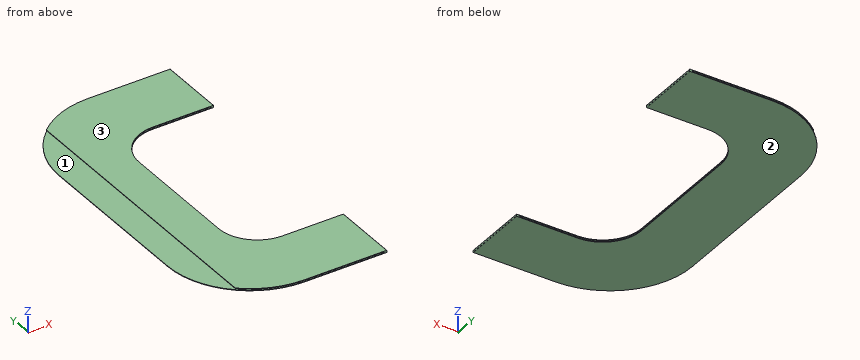
```python
from build123d import *

# Parameters (mm, degrees)
F1_DEPTH = 1.016
F2_W     = 160.02
F2_H     = 0.508
F3_DEPTH = 74.93
F4_W     = 34.701408
F4_H     = 184.597183
F5_DEPTH = 0.508
F6_R     = 0.254
F7_R     = 0.254
F9_DEPTH = 1.017


with BuildPart() as f1:
    # F0 (on Top) → F1 (new body)
    with BuildSketch(Plane.XY):
        with BuildLine():
            Line((0, -59.393544), (0, 93.006456))
            Line((0, 93.006456), (-38.1, 93.006456))
            ThreePointArc((-38.1, 93.006456), (-65.040768, 81.847225), (-76.2, 54.906456))
            Line((-76.2, 54.906456), (-76.2, -21.293544))
            ThreePointArc((-76.2, -21.293544), (-65.040768, -48.234312), (-38.1, -59.393544))
            Line((-38.1, -59.393544), (0, -59.393544))
        make_face()
    extrude(amount=F1_DEPTH)

    # F2 (on face) → F3 (cut)
    with BuildSketch(Plane(origin=(-76.2, 0, 0), x_dir=(0, -1, 0), z_dir=(-1, 0, 0))):
        with Locations((-18.385805, 0.508)):
            Rectangle(F2_W, F2_H)
    extrude(amount=-F3_DEPTH, mode=Mode.SUBTRACT)

    # F4 (on face) → F5 (cut)
    with BuildSketch(Plane.XY.offset(1.016)):
        with Locations((-80.850704, 13.036623)):
            Rectangle(F4_W, F4_H)
    extrude(amount=-F5_DEPTH, mode=Mode.SUBTRACT)

    # F6
    f6_edges = [f1.edges().sort_by_distance(p)[0] for p in [
        (0, 16.806456, 1.016),
    ]]
    fillet(f6_edges, radius=F6_R)

    # F7
    f7_edges = [f1.edges().sort_by_distance(p)[0] for p in [
        (0, 16.806456, 0),
    ]]
    fillet(f7_edges, radius=F7_R)

    # F8 (on face) → F9 (cut, through all)
    with BuildSketch(Plane.XY.offset(1.016)):
        with BuildLine():
            Line((40.75986, 62.526456), (-28.194, 62.526456))
            ThreePointArc((-28.194, 62.526456), (-40.766359, 57.318815), (-45.974, 44.746456))
            Line((-45.974, 44.746456), (-45.974, -11.133544))
            ThreePointArc((-45.974, -11.133544), (-40.766359, -23.705902), (-28.194, -28.913544))
            Line((-28.194, -28.913544), (40.75986, -28.913544))
            Line((40.75986, -28.913544), (40.75986, 62.526456))
        make_face()
    extrude(amount=-F9_DEPTH, mode=Mode.SUBTRACT)


solid = f1.part
```
For this review, take the finished solid that the model builds, in its own axes (mm). Face numbers are marked on the shaded views. Coordinates: 2 decimals unless noted, no trailing zeros. Write each loop counter-clockwise with the first axis right and the second up, starting at its lowest first coordinate (ties: lowest second). Pieces come first, ordered by that corner, then holes. Notation, with made-up numbers: (39.5, -28.5) -> (70.5, -28.5) arc R17 ccw to (70.5, -11.5) -> close; hole circle Ø6 at (27.25, 52). An arc over 180 degrees is marked (long way). Put each result on its own line as item: value.
Q1. The part is to be moulded in two halves that separate along Z. For the marked faces 1, 2 and 3, say which applies: +Z half, -Z half, draft (parallel to the pull), parting line (faces both ways), or undercut.
From the geometry:
face 1: undercut
face 2: -Z half
face 3: +Z half
Q2. Take a section at B-B, the plane x = -49. State the section outline as (y, z) points.
From the geometry:
outline: (-57.8, 0) -> (91.41, 0) -> (91.41, 0.25) -> (-57.8, 0.25) -> close; (-57.8, 0.76) -> (91.41, 0.76) -> (91.41, 1.02) -> (-57.8, 1.02) -> close
Q3. Take a section at D-D, the plane y = 66.5. State the section outline as (x, z) points.
From the geometry:
outline: (-74.39, 0) -> (-0.25, 0) arc R0.25 ccw to (0, 0.25) -> (0, 0.76) arc R0.25 ccw to (-0.25, 1.02) -> (-63.5, 1.02) -> (-63.5, 0.76) -> (-1.27, 0.76) -> (-1.27, 0.25) -> (-74.39, 0.25) -> close
Q4. Wall thickness on L1, parallel to Z at x = -56, y = -36; L2, parallel to Y at x = -8.5, z = 0.2; L3, parallel to X at y = 66, z = 0.5: over which ranges is each line inside the solid? List them lowest first.
From the geometry:
L1: z = 0 to 0.25, 0.76 to 1.02
L2: y = -59.39 to -28.91, 62.53 to 93.01
L3: x = -1.27 to 0
Q5. Take a section at C-C, the plane x = -33. State the section outline as (y, z) points.
From the geometry:
outline: (-59.39, 0) -> (-28.25, 0) -> (-28.25, 0.25) -> (-59.39, 0.25) -> close; (-59.39, 0.76) -> (-28.25, 0.76) -> (-28.25, 1.02) -> (-59.39, 1.02) -> close; (61.86, 0) -> (93.01, 0) -> (93.01, 0.25) -> (61.86, 0.25) -> close; (61.86, 0.76) -> (93.01, 0.76) -> (93.01, 1.02) -> (61.86, 1.02) -> close
Q6. Take a section at A-A, the plane y = 25. State the section outline as (x, z) points.
From the geometry:
outline: (-76.2, 0) -> (-45.97, 0) -> (-45.97, 0.25) -> (-76.2, 0.25) -> close; (-63.5, 0.76) -> (-45.97, 0.76) -> (-45.97, 1.02) -> (-63.5, 1.02) -> close
